Check sheet for the modelled part. Datum: model origin and axes. Units: mm. A direction names the side the tool comes from. Coordinates: 2 decimals unless noted, no trailing zeros. Loops run counter-clockwise (first coordinate to the right, second up) from the corner with the lowest first, then second, coordinate; pieces in that order, holes last. Notation, with made-up numbers: M -26,-20 L -1,-20 A31 cw -1,12 Z; hole C 79,-2 d2. An arc over 180 degrees is marked long. Use CSV: the item, a comma, the result in double quotes. Start each with the question number.
(1) Draft check along X on faces 4 (the cylindrical face through (14.583, 0.014, 18.5)), 5 (the flat face through (8, -8.1, 0.8)), 6 (the flat face through (9, 1, 17)), 7 (the cylindrical face through (7.417, 0.014, 23.5)). Enter one of: pulls with the +X half, pulls with the -X half, needs draft (parallel to the pull), parting line crosses it, or undercut.
(2) Section check C-C on x = 5. Record the cut outline in (y, z), and give its area (3 significant figures).
(3) Set-up check for faces 1 (the cylindrical face through (21.5, 0, 20.9)), 2 (the flat face through (14, 0, 16)), 3 (the flat face through (4, -14, 1)): record each of +Z, -Z, +X, -X, +Y, -Y from which the full face is reachable in a straight line by a thin tool's end or side.
(4) Scan lines: line 1 (X direction, y = -0.25, z = 21); line 2 (X direction, y = -20.75, z = 0.5); line 3 (Z direction, x = 1.5, y = -8.25). Record each from-to range of solid material in increasing order.
(5) Go/stop test with flat-tipped pins: pin 1 Ø2.5 at (x, y) = (4, -12.5) entering from +Z; pin 2 Ø11 at (y, z) = (-14.5, 7) entering from +X; pin 3 Ø1.6 at (x, y) = (12.5, 0.5) entering from -Z; pin 4 Ø1 at (x, z) = (6.5, 7.5) entering from -Y. Record where each tip stops, or that it passes through.
(6) Section check D-D on y = -10. Record the cut outline in (x, z), and give its area (3 significant figures).
(7) Section check A-A on z = 21. Record the cut outline in (x, y).
(8) Section check B-B on x = 17.25. Record the cut outline in (y, z), and give its area (3 significant figures).
from build123d import *

# Parameters (mm, degrees)
EXTRUDE_THIN1_DEPTH = 8
CHAMFER1_SIZE       = 6
SKETCH2_R           = 3.15
BOSS_EXTRUDE1_DEPTH = 2
SKETCH3_R           = 3.15
CUT_EXTRUDE1_DEPTH  = 10.6


with BuildPart() as part:
    # Sketch1 → Extrude-Thin1 (new body)
    with BuildSketch(Plane(origin=(0, 0, 0), x_dir=(0, 0, -1), z_dir=(1, 0, 0))):
        with BuildLine():
            Line((1, -25), (1, -3))
            ThreePointArc((1, -3), (-0.171572875, -0.171572875), (-3, 1))
            Line((-3, 1), (-21, 1))
            Line((-21, 1), (-21, -1))
            Line((-21, -1), (-3, -1))
            ThreePointArc((-3, -1), (-1.585786438, -1.585786438), (-1, -3))
            Line((-1, -3), (-1, -25))
            Line((-1, -25), (1, -25))
        make_face()
    extrude(amount=EXTRUDE_THIN1_DEPTH)

    # Chamfer1
    chamfer1_edges = [part.edges().sort_by_distance(p)[0] for p in [
        (0, 0, 21),
    ]]
    chamfer(chamfer1_edges, length=CHAMFER1_SIZE)

    # Sketch2 → Boss-Extrude1 (add)
    with BuildSketch(Plane(origin=(0, 1, 0), x_dir=(1, 0, 0), z_dir=(0, 1, 0))):
        with BuildLine():
            Line((0, -20.5), (0, -3))
            Line((0, -3), (8, -13))
            ThreePointArc((8, -13), (8.878679656, -15.121320344), (11, -16))
            Line((11, -16), (16.5, -16))
            ThreePointArc((16.5, -16), (21.5, -21), (16.5, -26))
            Line((16.5, -26), (5.5, -26))
            ThreePointArc((5.5, -26), (1.610912703, -24.389087297), (0, -20.5))
        make_face()
        with Locations(Location((16.5, -21, 0), (0, 0, 270))):
            Circle(SKETCH2_R, mode=Mode.SUBTRACT)
        with Locations((5.5, -21)):
            Circle(SKETCH2_R, mode=Mode.SUBTRACT)
    extrude(amount=-BOSS_EXTRUDE1_DEPTH)

    # Sketch3 → Cut-Extrude1 (cut)
    with BuildSketch(Plane(origin=(0, 1, 0), x_dir=(1, 0, 0), z_dir=(0, 1, 0))):
        with Locations(Location((5.5, -21, 0), (0, 0, 90))):
            Circle(SKETCH3_R)
    extrude(amount=-CUT_EXTRUDE1_DEPTH, mode=Mode.SUBTRACT)


solid = part.part
Outcome:
1,face 4,"undercut"
1,face 5,"pulls with the +X half"
1,face 6,"needs draft"
1,face 7,"undercut"
2,outline,"M -25,-1 L -3,-1 A4 ccw 1,3 L 1,17.89 L -1,17.89 L -1,3 A2 cw -3,1 L -25,1 Z; M -1,24.11 L 1,24.11 L 1,25.98 L -1,25.98 Z"
2,area,"86.9 mm²"
3,face 1,"+X, +Y, -Y"
3,face 2,"-Z, +X, +Y, -Y"
3,face 3,"+Z, +X, -X, -Y"
4,line 1,"x = 0.02 to 2.35, 8.65 to 13.35, 19.65 to 21.5"
4,line 2,"x = 0 to 8"
4,line 3,"z = -1 to 1"
5,pin 1,"stops at z = 1"
5,pin 2,"passes through"
5,pin 3,"stops at z = 16"
5,pin 4,"stops at y = -1"
6,outline,"M 0,-1 L 8,-1 L 8,1 L 0,1 Z"
6,area,"16.0 mm²"
7,outline,"M 0.02,-1 L 2.35,-1 L 2.35,1 L 0.02,1 Z; M 8.65,-1 L 13.35,-1 L 13.35,1 L 8.65,1 Z; M 19.65,-1 L 21.5,-1 L 21.5,1 L 19.65,1 Z"
8,outline,"M -1,16.06 L 1,16.06 L 1,17.94 L -1,17.94 Z; M -1,24.06 L 1,24.06 L 1,25.94 L -1,25.94 Z"
8,area,"7.54 mm²"
